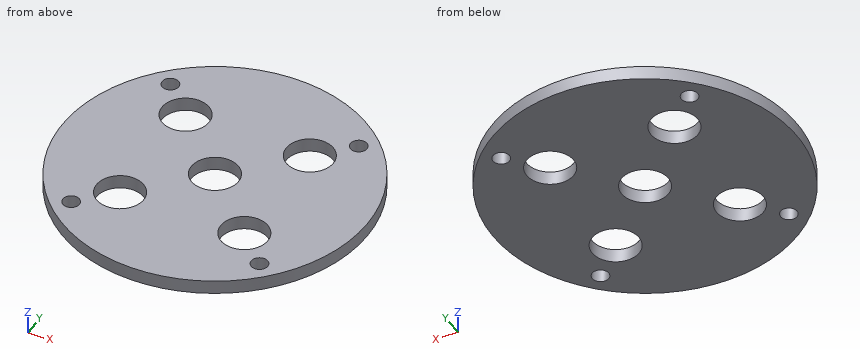
```python
from build123d import *

# Parameters (mm, degrees)
SKETCH2_R           = 11
SKETCH2_R_2         = 1.7
SKETCH2_R_3         = 0.6
BOSS_EXTRUDE1_DEPTH = 1


with BuildPart() as part:
    # Sketch2 → Boss-Extrude1 (new body)
    with BuildSketch(Plane.XY):
        with Locations((0, -8.8655e-05)):
            Circle(SKETCH2_R)
        with Locations((-4.490128061, 4.490039406)):
            Circle(SKETCH2_R_2, mode=Mode.SUBTRACT)
        with Locations((4.490128061, 4.490039406)):
            Circle(SKETCH2_R_2, mode=Mode.SUBTRACT)
        with Locations((-4.490128061, -4.490216715)):
            Circle(SKETCH2_R_2, mode=Mode.SUBTRACT)
        with Locations((4.490128061, -4.490216715)):
            Circle(SKETCH2_R_2, mode=Mode.SUBTRACT)
        with Locations((0, -8.8655e-05)):
            Circle(SKETCH2_R_2, mode=Mode.SUBTRACT)
        with Locations((6.80553822, 6.805449565)):
            Circle(SKETCH2_R_3, mode=Mode.SUBTRACT)
        with Locations((6.805449565, -6.80553822)):
            Circle(SKETCH2_R_3, mode=Mode.SUBTRACT)
        with Locations((-6.80553822, -6.805449565)):
            Circle(SKETCH2_R_3, mode=Mode.SUBTRACT)
        with Locations((-6.805449565, 6.80553822)):
            Circle(SKETCH2_R_3, mode=Mode.SUBTRACT)
    extrude(amount=BOSS_EXTRUDE1_DEPTH)


solid = part.part
```
CAD build for the part. Positions are in the model's coordinates, mm. Round coordinates to 2 decimals unless told otherwise and drop trailing zeros. Order: outer loops, then holes, each group sorted by start corner. A loop starts at its lowest first (then second) coordinate and runs counter-clockwise, first axis right, second up.
Item 1: Saw through at D-D on z = 0.6. State how many separate pieces and enclosed holes the cut face has, then the cut area to 3 significant figures.
Item 2: Saw through at C-C on x = 3.75. Write the cut outline in (y, z), then the cut area to 3 significant figures.
Item 3: Pin check, flat tips, straight feed: pin 1 (1.4 mm diameter, centred on x = -6.81, y = 6.81, fed in from -Z); pin 2 (2 mm diameter, centred on x = -4.49, y = -4.49, fed in from +Z). Stop position of each tip, or through.
Item 4: Probe line 1 along X through (y, z) = (4.25, 0.45); line 2 along Y through (x, z) = (-3, 0.8); line 3 along X through (y, z) = (-4.75, 0.3). List the from-to ranges inside material, lowest first.
Item 5: Saw through at B-B on y = 1. Write the cut outline in (x, z), then the cut area to 3 significant figures.
Item 6: Saw through at A-A on x = 0. Write the cut outline in (y, z), then the cut area to 3 significant figures.
Reported:
1. separate pieces: 1
1. enclosed holes: 9
1. area: 330 mm2
2. outline: (-10.34, 0) - (-6.02, 0) - (-6.02, 1) - (-10.34, 1) - close; (-2.96, 0) - (2.96, 0) - (2.96, 1) - (-2.96, 1) - close; (6.02, 0) - (10.34, 0) - (10.34, 1) - (6.02, 1) - close
2. area: 14.6 mm2
3. pin 1: stops at z = 0
3. pin 2: passes through
4. line 1: x = -10.15 to -6.17, -2.81 to 2.81, 6.17 to 10.15
4. line 2: y = -10.58 to -5.31, -3.67 to 3.67, 5.31 to 10.58
4. line 3: x = -9.92 to -6.17, -2.81 to 2.81, 6.17 to 9.92
5. outline: (-10.95, 0) - (-1.37, 0) - (-1.37, 1) - (-10.95, 1) - close; (1.37, 0) - (10.95, 0) - (10.95, 1) - (1.37, 1) - close
5. area: 19.2 mm2
6. outline: (-11, 0) - (-1.7, 0) - (-1.7, 1) - (-11, 1) - close; (1.7, 0) - (11, 0) - (11, 1) - (1.7, 1) - close
6. area: 18.6 mm2
